Build history of the part. All positions in model axes, mm. Give positions to 0.01 mm unless a question says otherwise; leave off trailing zeros. Order: outer loops, then holes, each group sorted by start corner. A loop starts at its lowest first (then second) coordinate and runs counter-clockwise, first axis right, second up. Notation, with made-up numbers: (67, 20) - (86, 20) arc R20 cw to (86, 59) - close; hole circle Ø2 at (-13, 66.5). An arc over 180 degrees is marked (long way). Answer in a Markdown table with one row per item.
```python
from build123d import *

# Parameters (mm, degrees)
SKETCH1_R                   = 35
BOSS_EXTRUDE1_DEPTH         = 100
SKETCH2_R                   = 2.5
CUT_EXTRUDE5_DEPTH          = 15
SKETCH2_7_R                 = 25
CUT_EXTRUDE6_DEPTH          = 10
SKETCH3_R                   = 10
CUT_EXTRUDE8_DEPTH          = 112.579568022
F_1_4_20_TAPPED_HOLE1_D     = 5.1054
F_1_4_20_TAPPED_HOLE1_DEPTH = 19.1
F_1_4_20_TAPPED_HOLE1_TIP   = 1.533816902


with BuildPart() as part:
    # Sketch1 → Boss-Extrude1 (new body)
    with BuildSketch(Plane.XY):
        Circle(SKETCH1_R)
    extrude(amount=BOSS_EXTRUDE1_DEPTH)

    # Sketch2 → Cut-Extrude5 (cut)
    with BuildSketch(Plane.XY.offset(100)):
        with Locations((0, 20)):
            Circle(SKETCH2_R)
        with Locations((8.134732862, 18.270909153)):
            Circle(SKETCH2_R)
        with Locations((14.86289651, 13.382612127)):
            Circle(SKETCH2_R)
        with Locations((19.021130326, 6.180339887)):
            Circle(SKETCH2_R)
        with Locations((19.890437907, -2.090569265)):
            Circle(SKETCH2_R)
        with Locations((17.320508076, -10)):
            Circle(SKETCH2_R)
        with Locations((11.755705046, -16.180339887)):
            Circle(SKETCH2_R)
        with Locations((4.158233816, -19.562952015)):
            Circle(SKETCH2_R)
        with Locations((-4.158233816, -19.562952015)):
            Circle(SKETCH2_R)
        with Locations((-11.755705046, -16.180339887)):
            Circle(SKETCH2_R)
        with Locations((-17.320508076, -10)):
            Circle(SKETCH2_R)
        with Locations((-19.890437907, -2.090569265)):
            Circle(SKETCH2_R)
        with Locations((-19.021130326, 6.180339887)):
            Circle(SKETCH2_R)
        with Locations((-14.86289651, 13.382612127)):
            Circle(SKETCH2_R)
        with Locations((-8.134732862, 18.270909153)):
            Circle(SKETCH2_R)
    extrude(amount=-CUT_EXTRUDE5_DEPTH, mode=Mode.SUBTRACT)

    # Sketch2<7> → Cut-Extrude6 (cut)
    with BuildSketch(Plane.XY.offset(100)):
        Circle(SKETCH2_7_R)
    extrude(amount=-CUT_EXTRUDE6_DEPTH, mode=Mode.SUBTRACT)

    # Sketch3 → Cut-Extrude8 (cut, through all)
    with BuildSketch(Plane.XY):
        Circle(SKETCH3_R)
    extrude(amount=CUT_EXTRUDE8_DEPTH, mode=Mode.SUBTRACT)

    # 1/4-20 Tapped Hole1
    with Locations(Plane(origin=(0.951346155, -34.987068189, 51.695877928), x_dir=(-0.999630519699, -0.027181318711, 0), z_dir=(0.027181318711, -0.999630519699, 0))):
        with Locations((0, 0)):
            Hole(F_1_4_20_TAPPED_HOLE1_D / 2, depth=F_1_4_20_TAPPED_HOLE1_DEPTH)
            with Locations((0, 0, -(F_1_4_20_TAPPED_HOLE1_DEPTH + F_1_4_20_TAPPED_HOLE1_TIP / 2))):  # 118° drill point
                Cone(0, F_1_4_20_TAPPED_HOLE1_D / 2, F_1_4_20_TAPPED_HOLE1_TIP, mode=Mode.SUBTRACT)


solid = part.part
```
1. Cut at C-C on x = -28. Write the cut outline in (y, z).
Check result:
| item | result |
|---|---|
| outline | (-21, 0) - (21, 0) - (21, 100) - (-21, 100) - close |
2. Drop flat-ended pins along their axis: P1, Ø5.5, axis at x = 21, y = -2, coming from the +Z side; P2, Ø10, axis at x = 18, z = 24.5, coming from the -Y side; P3, Ø2.5, axis at x = 4, y = -18.5, coming from the +Z side; P4, Ø6, axis at x = -18.5, y = 14, coming from the -Z side. Give the stop position or say it passes through.
Check result:
| item | result |
|---|---|
| P1 | stops at z = 90 |
| P2 | stops at y = -32.5 |
| P3 | stops at z = 85 |
| P4 | stops at z = 0 |
3. Cut at B-B on z = 83.5. Write the cut outline in (x, y), and give its area (3 significant figures).
Check result:
| item | result |
|---|---|
| outline | circle Ø70 at (0, 0); hole circle Ø20 at (0, 0) |
| area | 3,530 mm² |
4. Cut at D-D on x = 27.5. Write the cut outline in (y, z).
Check result:
| item | result |
|---|---|
| outline | (-21.65, 0) - (21.65, 0) - (21.65, 100) - (-21.65, 100) - close |
5. Probe line 1 (Y direction, x = -11.5, z = 87); line 2 (Z direction, x = 13, y = 12.5); line 3 (Z direction, x = 21.5, y = -11.5). List the from-to ranges inside material, lowest first.
Check result:
| item | result |
|---|---|
| line 1 | y = -33.06 to -18.67, -13.69 to 33.06 |
| line 2 | z = 0 to 85 |
| line 3 | z = 0 to 90 |
6. Cut at A-A on y = 5. Write the cut outline in (x, z), and give its area (3 significant figures).
Check result:
| item | result |
|---|---|
| outline | (-34.64, 0) - (-8.66, 0) - (-8.66, 90) - (-16.82, 90) - (-16.82, 85) - (-21.22, 85) - (-21.22, 90) - (-24.49, 90) - (-24.49, 100) - (-34.64, 100) - close; (8.66, 0) - (34.64, 0) - (34.64, 100) - (24.49, 100) - (24.49, 90) - (21.22, 90) - (21.22, 85) - (16.82, 85) - (16.82, 90) - (8.66, 90) - close |
| area | 4,840 mm² |
7. Two-plate mould, pull along Y, no slides. Class faces 1 (the face through (-12.55, 12.43, 87.54)), 2 (the face through (-28, -21, 49)): +Y half, -Y half, draft (parallel to the pull), parting line (faces both ways), or undercut.
Check result:
| item | result |
|---|---|
| face 1 | undercut |
| face 2 | parting line |
